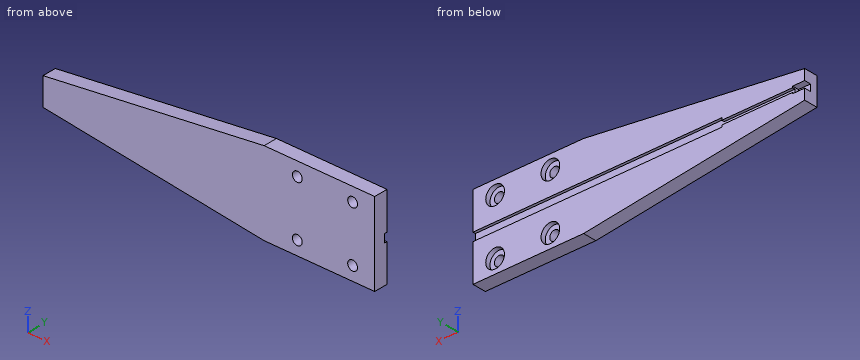
from build123d import *

# Parameters (mm, degrees)
SKETCH2_W                       = 38.1
SKETCH2_H                       = 6.35
BOSS_EXTRUDE1_DEPTH             = 152.4
CBORE_FOR_M4_SBHCS1_D           = 4.5
CBORE_FOR_M4_SBHCS1_CBORE_D     = 8.6
CBORE_FOR_M4_SBHCS1_CBORE_DEPTH = 2.2
SKETCH9_W                       = 3.048
SKETCH9_H                       = 3.048
CUT_EXTRUDE1_DEPTH              = 5.588
SKETCH12_W                      = 114.3
SKETCH12_H                      = 3.81
CUT_EXTRUDE2_DEPTH              = 1.27
SKETCH13_W                      = 32.512
SKETCH13_H                      = 1.905
CUT_EXTRUDE3_DEPTH              = 1.27
CUT_EXTRUDE4_DEPTH              = 6.35
CUT_EXTRUDE5_DEPTH              = 6.35


with BuildPart() as part:
    # Sketch2 → Boss-Extrude1 (new body)
    with BuildSketch(Plane(origin=(0, 0, 0), x_dir=(0, 0, -1), z_dir=(1, 0, 0))):
        Rectangle(SKETCH2_W, SKETCH2_H)
    extrude(amount=BOSS_EXTRUDE1_DEPTH)

    # CBORE for M4 SBHCS1 (through all)
    with Locations(Plane(origin=(0, 3.175, 0), x_dir=(1, 0, 0), z_dir=(0, 1, 0))):
        with Locations((142.247626007, -12.7), (142.247626007, 12.7), (116.847626007, 12.7), (116.847626007, -12.7)):
            CounterBoreHole(CBORE_FOR_M4_SBHCS1_D / 2, CBORE_FOR_M4_SBHCS1_CBORE_D / 2, CBORE_FOR_M4_SBHCS1_CBORE_DEPTH)

    # Sketch9 → Cut-Extrude1 (cut)
    with BuildSketch(Plane.ZY):
        with Locations((0, 1.651)):
            Rectangle(SKETCH9_W, SKETCH9_H)
    extrude(amount=-CUT_EXTRUDE1_DEPTH, mode=Mode.SUBTRACT)

    # Sketch12 → Cut-Extrude2 (cut)
    with BuildSketch(Plane(origin=(0, 3.175, 0), x_dir=(1, 0, 0), z_dir=(0, 1, 0))):
        with Locations((95.25, 0)):
            Rectangle(SKETCH12_W, SKETCH12_H)
    extrude(amount=-CUT_EXTRUDE2_DEPTH, mode=Mode.SUBTRACT)

    # Sketch13 → Cut-Extrude3 (cut)
    with BuildSketch(Plane(origin=(0, 3.175, 0), x_dir=(1, 0, 0), z_dir=(0, 1, 0))):
        with Locations((21.844, 0.0635)):
            Rectangle(SKETCH13_W, SKETCH13_H)
    extrude(amount=-CUT_EXTRUDE3_DEPTH, mode=Mode.SUBTRACT)

    # Sketch14 → Cut-Extrude4 (cut)
    with BuildSketch(Plane(origin=(0, 3.175, 0), x_dir=(1, 0, 0), z_dir=(0, 1, 0))):
        Polygon((0, 6.35), (0, 19.05), (101.6, 19.05), align=None)
    extrude(amount=-CUT_EXTRUDE4_DEPTH, mode=Mode.SUBTRACT)

    # Sketch15 → Cut-Extrude5 (cut)
    with BuildSketch(Plane(origin=(0, 3.175, 0), x_dir=(1, 0, 0), z_dir=(0, 1, 0))):
        Polygon((0, -6.35), (101.6, -19.05), (0, -19.05), align=None)
    extrude(amount=-CUT_EXTRUDE5_DEPTH, mode=Mode.SUBTRACT)


solid = part.part
The listing builds one solid part. Answer for the finished solid, in the listing's coordinates (mm). Give positions to 0.01 mm unless a question says otherwise; leave off trailing zeros. Write each loop counter-clockwise with the first axis right and the second up, starting at its lowest first coordinate (ties: lowest second). Pieces come first, ordered by that corner, then holes. Notation, with made-up numbers: (86.5, 21.5) -> (134.5, 21.5) arc R30 cw to (134.5, 52.5) -> close; hole circle Ø5 at (64.5, -15). An arc over 180 degrees is marked (long way). Use a Markdown table: item, result.
(1) Section D-D, the plane x = 84.5 is taken. Determine the outline of the cut face in (y, z) (1 decimal), then the cut area to 3 significant figures.
Return value:
| item | result |
|---|---|
| outline | (-3.2, -16.9) -> (3.2, -16.9) -> (3.2, -1.9) -> (1.9, -1.9) -> (1.9, 1.9) -> (3.2, 1.9) -> (3.2, 16.9) -> (-3.2, 16.9) -> close |
| area | 210 mm2 |
(2) Section A-A, the plane z = 12.7 is taken. Determine the outline of the cut face in (x, y) (3 decimals).
Return value:
| item | result |
|---|---|
| outline | (50.8, -3.175) -> (114.598, -3.175) -> (114.598, 0.975) -> (112.548, 0.975) -> (112.548, 3.175) -> (50.8, 3.175) -> close; (119.098, -3.175) -> (139.998, -3.175) -> (139.998, 0.975) -> (137.948, 0.975) -> (137.948, 3.175) -> (121.148, 3.175) -> (121.148, 0.975) -> (119.098, 0.975) -> close; (144.498, -3.175) -> (152.4, -3.175) -> (152.4, 3.175) -> (146.548, 3.175) -> (146.548, 0.975) -> (144.498, 0.975) -> close |
(3) Section C-C, the plane x = 127 is taken. Determine the outline of the cut face in (y, z) (3 decimals).
Return value:
| item | result |
|---|---|
| outline | (-3.175, -19.05) -> (3.175, -19.05) -> (3.175, -1.905) -> (1.905, -1.905) -> (1.905, 1.905) -> (3.175, 1.905) -> (3.175, 19.05) -> (-3.175, 19.05) -> close |
(4) Flat-ended cylindrical pins translate along their axes: P1, Ø1, axis at x = 27, y = 2.5, coming from the -Z side; P2, Ø1.5, axis at y = 2, z = 0.5, coming from the -X side; P3, Ø7, axis at x = 116.85, z = 12.7, coming from the +Y side (3 decimals). Find the tip coordinate at first contact, or state that the pin passes through.
Return value:
| item | result |
|---|---|
| P1 | z = -9.79 |
| P2 | x = 5.59 |
| P3 | y = 0.975 |
(5) Section B-B, the plane y = -1.5 is taken. Determine the outline of the cut face in (x, z).
Return value:
| item | result |
|---|---|
| outline | (0, -6.35) -> (101.6, -19.05) -> (152.4, -19.05) -> (152.4, 19.05) -> (101.6, 19.05) -> (0, 6.35) -> close; hole circle Ø4.5 at (116.85, -12.7); hole circle Ø4.5 at (116.85, 12.7); hole circle Ø4.5 at (142.25, -12.7); hole circle Ø4.5 at (142.25, 12.7) |
(6) Find the intervals of material crossed by probe 1 along Z at (x, y) = (140.5, -1); probe 2 along Z at (x, y) = (30.5, 2.75); probe 3 along Y at (x, z) = (99, -1) (3 decimals), in increasing order. Write a range as from..to.
Return value:
| item | result |
|---|---|
| probe 1 | -19.05..-14.12, -11.28..11.28, 14.12..19.05 |
| probe 2 | -10.16..-1.02, 0.89..10.16 |
| probe 3 | -3.175..1.905 |
